Design review of the part built by this model. Coordinates are the model's own, in mm. Face numbers are marked on the shaded views. Give positions to 0.01 mm unless a question says otherwise; leave off trailing zeros. Loops run counter-clockwise (first coordinate to the right, second up) from the corner with the lowest first, then second, coordinate; pieces in that order, holes last. Notation, with made-up numbers: (47.5, -15) - (76.5, -15) arc R9 cw to (76.5, -7) - close; hole circle Ø4 at (78, -22). An arc over 180 degrees is marked (long way). One line per item, written item: value. Start each with the question number.
```python
from build123d import *

# Parameters (mm, degrees)
ESBO_O1_R                = 15
ESBO_O1_R_2              = 7
ESBO_O1_R_3              = 1.25
RESSALTO_EXTRUS_O1_DEPTH = 7


with BuildPart() as part:
    # Esboço1 → Ressalto-extrusão1 (new, symmetric)
    with BuildSketch(Plane.XY):
        Circle(ESBO_O1_R)
        Circle(ESBO_O1_R_2, mode=Mode.SUBTRACT)
        with Locations((0, 11)):
            Circle(ESBO_O1_R_3, mode=Mode.SUBTRACT)
        with Locations((7.778174593, 7.778174593)):
            Circle(ESBO_O1_R_3, mode=Mode.SUBTRACT)
        with Locations((11, 0)):
            Circle(ESBO_O1_R_3, mode=Mode.SUBTRACT)
        with Locations((7.778174593, -7.778174593)):
            Circle(ESBO_O1_R_3, mode=Mode.SUBTRACT)
        with Locations((0, -11)):
            Circle(ESBO_O1_R_3, mode=Mode.SUBTRACT)
        with Locations((-7.778174593, -7.778174593)):
            Circle(ESBO_O1_R_3, mode=Mode.SUBTRACT)
        with Locations((-11, 0)):
            Circle(ESBO_O1_R_3, mode=Mode.SUBTRACT)
        with Locations((-7.778174593, 7.778174593)):
            Circle(ESBO_O1_R_3, mode=Mode.SUBTRACT)
    extrude(amount=RESSALTO_EXTRUS_O1_DEPTH, both=True)


solid = part.part
```
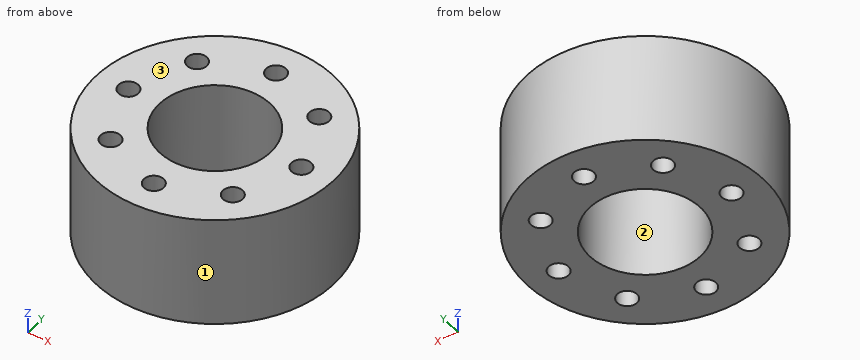
(1) To check wall thickness, follow L1, parallel to Y at x = 0, z = -1; L2, parallel to X at y = -8.25, z = 5.5; L3, parallel to Y at x = 8, z = -2. State the ranges of each line that lie inside material, in increasing order. Write a range as from..to.
(2) For pin 1 Ø3 at (x, y) = (7.78, -7.78) entering from -Z; pin 2 Ø1.5 at (y, z) = (6.5, -1) entering from +X; pin 3 Ø6 at (y, z) = (-12, -1) entering from +X; pin 4 Ø3 at (y, z) = (-5.5, -2) entering from -X, all flat-tipped, find the tip position at first contact; note any pin that passes through.
(3) Take a section at D-D on x = 11. State the section outline as (y, z) points.
(4) Take a section at A-A on y = 5.25. State the section outline as (x, z) points.
(5) Take a section at B-B on x = 0. State the section outline as (y, z) points, and give its area (3 significant figures).
(6) Draft analysis for pull direction Y (two halves, no side actions). For the marked faces 1, 2 and 3, state which applies: pulls with the +Y half, pulls with the -Y half, needs draft (parallel to the pull), parting line crosses it, or undercut.
Here are the results:
1. L1: -15..-12.25, -9.75..-7, 7..9.75, 12.25..15
1. L2: -12.53..-8.94, -6.62..6.62, 8.94..12.53
1. L3: -12.69..-9.01, -6.55..6.55, 9.01..12.69
2. pin 1: z = -7
2. pin 2: x = 13.85
2. pin 3: x = 12
2. pin 4: x = -14.46
3. outline: (-10.2, -7) - (-1.25, -7) - (-1.25, 7) - (-10.2, 7) - close; (1.25, -7) - (10.2, -7) - (10.2, 7) - (1.25, 7) - close
4. outline: (-14.05, -7) - (-4.63, -7) - (-4.63, 7) - (-14.05, 7) - close; (4.63, -7) - (14.05, -7) - (14.05, 7) - (4.63, 7) - close
5. outline: (-15, -7) - (-12.25, -7) - (-12.25, 7) - (-15, 7) - close; (-9.75, -7) - (-7, -7) - (-7, 7) - (-9.75, 7) - close; (7, -7) - (9.75, -7) - (9.75, 7) - (7, 7) - close; (12.25, -7) - (15, -7) - (15, 7) - (12.25, 7) - close
5. area: 154 mm²
6. face 1: parting line crosses it
6. face 2: undercut
6. face 3: needs draft
